Geometry check sheet. Reference: the model listing, model coordinates, mm. Give positions to 0.01 mm unless a question says otherwise; leave off trailing zeros. Order: outer loops, then holes, each group sorted by start corner. A loop starts at its lowest first (then second) coordinate and runs counter-clockwise, first axis right, second up.
from build123d import *


with BuildPart() as part:
    # Sketch2 → Revolve1 (revolve)
    with BuildSketch(Plane(origin=(0, 0, 0), x_dir=(0, 0, -1), z_dir=(1, 0, 0))):
        with BuildLine():
            Line((0, 3), (0, 5))
            Line((0, 5), (-0.2, 5))
            ThreePointArc((-0.2, 5), (-0.5, 4.783772234), (-0.8, 5))
            Line((-0.8, 5), (-1, 5))
            Line((-1, 5), (-1, 3))
            Line((-1, 3), (0, 3))
        make_face()
    revolve1 = revolve(axis=Axis((0, 0, 3.014677367), (0, 0, -1)))

    # Mirror2: Revolve1 across plane
    add(revolve1.mirror(Plane(origin=(0, 0, 0), x_dir=(1, 0, 0), z_dir=(0, 0, -1))))


solid = part.part
Item 1: Sectioned sample at D-D (z = 0.65). Enter the section's corners in (x, y).
Reported:
outline: circle Ø9.64 at (0, 0); hole circle Ø6 at (0, 0)
Item 2: Scan lines: L1, parallel to X at y = -2.5, z = -0.15; L2, parallel to X at y = 0, z = 0.65; L3, parallel to Y at x = 2.75, z = 0.35. Record each from-to range of solid material in increasing order.
Reported:
L1: x = -4.33 to -1.66, 1.66 to 4.33
L2: x = -4.82 to -3, 3 to 4.82
L3: y = -3.96 to -1.2, 1.2 to 3.96
Item 3: Gauge pin test, flat end, axial feed: pin 1 (3.5 mm diameter, centred on x = 0, y = 0, fed in from -Z). Record the tip position at first contact, or that the pin passes through.
Reported:
pin 1: passes through
Item 4: Sectioned sample at C-C (z = -0.6). Enter the section's corners in (x, y), and give its area (3 significant figures).
Reported:
outline: circle Ø9.6 at (0, 0); hole circle Ø6 at (0, 0)
area: 44.1 mm2
Item 5: Sectioned sample at A-A (x = 0). Enter the section's corners in (y, z), and give its area (3 significant figures).
Reported:
outline: (-5, -1) - (-3, -1) - (-3, 1) - (-5, 1) - (-5, 0.8) arc R0.32 cw to (-5, 0.2) - (-5, -0.2) arc R0.32 cw to (-5, -0.8) - close; (3, -1) - (5, -1) - (5, -0.8) arc R0.32 cw to (5, -0.2) - (5, 0.2) arc R0.32 cw to (5, 0.8) - (5, 1) - (3, 1) - close
area: 7.62 mm2
